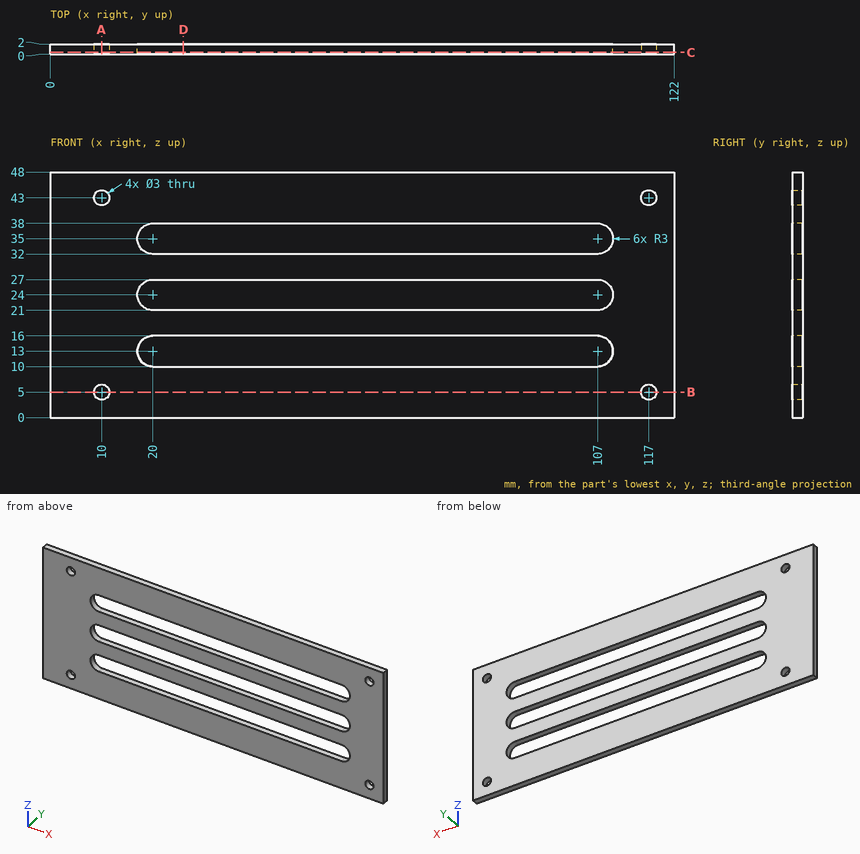
Here's the drawing with two shaded views (mm, measured from the low corner). I have some questions. Coordinates: 2 decimals unless noted, no trailing zeros. Write each loop counter-clockwise with the first axis right and the second up, starting at its lowest first coordinate (ties: lowest second). Pieces come first, ordered by that corner, then holes. Notation, with made-up numbers: M 41,77.25 L 71,77.25 A15 cw 71,102.25 Z; hole C 6.25,-38 d9. An arc over 180 degrees is marked long. Use one line per item in the form item = value.
Q1. If we section it at A-A (x = 10): Write out the boundary of the cut face in (y, z), then the cut area to 3 significant figures.
Model answer:
outline = M 0,0 L 2,0 L 2,3.5 L 0,3.5 Z; M 0,6.5 L 2,6.5 L 2,41.5 L 0,41.5 Z; M 0,44.5 L 2,44.5 L 2,48 L 0,48 Z
area = 84.0 mm^2
Q2. If we section it at D-D (x = 26): Write out the boundary of the cut face in (y, z), then the cut area to 3 significant figures.
Model answer:
outline = M 0,0 L 2,0 L 2,10 L 0,10 Z; M 0,16 L 2,16 L 2,21 L 0,21 Z; M 0,27 L 2,27 L 2,32 L 0,32 Z; M 0,38 L 2,38 L 2,48 L 0,48 Z
area = 60.0 mm^2
Q3. If we section it at B-B (z = 5): Write out the boundary of the cut face in (x, y), then the cut area to 3 significant figures.
Model answer:
outline = M 0,0 L 8.5,0 L 8.5,2 L 0,2 Z; M 11.5,0 L 115.5,0 L 115.5,2 L 11.5,2 Z; M 118.5,0 L 122,0 L 122,2 L 118.5,2 Z
area = 232 mm^2
Q4. If we section it at C-C (y = 0.35): Write out the boundary of the cut face in (x, z).
Model answer:
outline = M 0,0 L 122,0 L 122,48 L 0,48 Z; hole C 10,5 d3; hole C 10,43 d3; hole M 20,10 L 107,10 A3 ccw 107,16 L 20,16 A3 ccw Z; hole M 20,21 L 107,21 A3 ccw 107,27 L 20,27 A3 ccw Z; hole M 20,32 L 107,32 A3 ccw 107,38 L 20,38 A3 ccw Z; hole C 117,5 d3; hole C 117,43 d3
Q5. For P1, Ø1.8, axis at x = 10, z = 5, coming from the +Y side, with a flat end and sliding along its axis, tell me the tip position at first contact or that it passes through.
Model answer:
P1 = through
Q6. I need wall thicknesses on line 1 along X through (y, z) = (1.6, 5); line 2 along Z through (x, y) = (56, 1.25); line 3 along X through (y, z) = (1.05, 35). Which ranges of each line are inside material? Lowest first, please. Write a range as from..to.
Model answer:
line_1 = 0..8.5, 11.5..115.5, 118.5..122
line_2 = 0..10, 16..21, 27..32, 38..48
line_3 = 0..17, 110..122
